from build123d import *

# Parameters (mm, degrees)
SKETCH2_W                = 13
SKETCH2_H                = 21
SKETCH2_W_2              = 12
SKETCH2_H_2              = 20
BOSS_EXTRUDE1_DEPTH      = 3
SKETCH2_2_W              = 12
SKETCH2_2_H              = 20
BOSS_EXTRUDE2_DEPTH      = 3
BOSS_EXTRUDE2_DEPTH_BACK = 5
SKETCH3_W                = 7.910089125
SKETCH3_H                = 16.025972414
SKETCH3_W_2              = 7.710089125
SKETCH3_H_2              = 15.825972414
CUT_EXTRUDE1_DEPTH       = 3
SKETCH3_2_W              = 7.710089125
SKETCH3_2_H              = 15.825972414
BOSS_EXTRUDE3_DEPTH      = 3
CUT_EXTRUDE2_DEPTH       = 11.644897537


with BuildPart() as part:
    # Sketch2 → Boss-Extrude1 (new body)
    with BuildSketch(Plane(origin=(0, 0, 0), x_dir=(1, 0, 0), z_dir=(0, 1, 0))):
        with Locations((-0.268196817, 0.402295225)):
            Rectangle(SKETCH2_W, SKETCH2_H)
        with Locations((-0.268196817, 0.402295225)):
            Rectangle(SKETCH2_W_2, SKETCH2_H_2, mode=Mode.SUBTRACT)
    extrude(amount=BOSS_EXTRUDE1_DEPTH)

    # Sketch2_2 → Boss-Extrude2 (add, two sides)
    with BuildSketch(Plane(origin=(0, 0, 0), x_dir=(1, 0, 0), z_dir=(0, 1, 0))) as boss_extrude2_sk:
        with Locations((-0.268196817, 0.402295225)):
            Rectangle(SKETCH2_2_W, SKETCH2_2_H)
    extrude(amount=BOSS_EXTRUDE2_DEPTH)
    extrude(boss_extrude2_sk.sketch, amount=-BOSS_EXTRUDE2_DEPTH_BACK)

    # Sketch3 → Cut-Extrude1 (cut)
    with BuildSketch(Plane(origin=(0, 3, 0), x_dir=(1, 0, 0), z_dir=(0, 1, 0))):
        with Locations((0.021656158, 0.039979007)):
            Rectangle(SKETCH3_W, SKETCH3_H)
        with Locations((0.021656157, 0.039979007)):
            Rectangle(SKETCH3_W_2, SKETCH3_H_2, mode=Mode.SUBTRACT)
    extrude(amount=-CUT_EXTRUDE1_DEPTH, mode=Mode.SUBTRACT)

    # Sketch3_2 → Boss-Extrude3 (add)
    with BuildSketch(Plane(origin=(0, 3, 0), x_dir=(1, 0, 0), z_dir=(0, 1, 0))):
        with Locations((0.021656157, 0.039979007)):
            Rectangle(SKETCH3_2_W, SKETCH3_2_H)
    extrude(amount=BOSS_EXTRUDE3_DEPTH)

    # Sketch5 → Cut-Extrude2 (cut, through all)
    with BuildSketch(Plane(origin=(3.87670072, 0, 0), x_dir=(0, 0, -1), z_dir=(1, 0, 0))):
        with BuildLine():
            add(Edge.make_bspline(
                [(7.952965214, 3.003696013), (-0.44948354, 3.292111909), (-7.8730072, 5.997516068)],
                knots=[0.001628514, 0.001628514, 0.001628514, 0.990717924, 0.990717924, 0.990717924], degree=2))
            Line((7.952965214, 3.003696013), (7.952965214, 6))
            Line((7.952965214, 6), (-7.8730072, 6))
            Line((-7.8730072, 6), (-7.8730072, 5.997516068))
        make_face()
    extrude(amount=-CUT_EXTRUDE2_DEPTH, mode=Mode.SUBTRACT)


solid = part.part
Source: CAD feature listing. Evaluate the final solid. Frame: model axes, mm. A direction names the side the tool comes from. Give positions to 0.01 mm unless a question says otherwise; leave off trailing zeros. Write each loop counter-clockwise with the first axis right and the second up, starting at its lowest first coordinate (ties: lowest second). Pieces come first, ordered by that corner, then holes. Notation, with made-up numbers: (-36, 2.25) -> (23, 2.25) arc R14 ccw to (23, 21.25) -> close; hole circle Ø1 at (63.25, -8). An arc over 180 degrees is marked (long way). Write item = value, one per line.
Q1. First-contact query: pin 1 (1.5 mm diameter, centred on y = -1.5, z = 0.5, fed in from +X); pin 2 (1 mm diameter, centred on y = -2.5, z = 7.5, fed in from -X); pin 3 (4 mm diameter, centred on x = -1, z = -0.5, fed in from +Y). Flat tips, straight axial feed; report the tip coordinate or a pass-through.
Here are the results:
pin_1 = 5.73
pin_2 = -6.27
pin_3 = 4.16
Q2. Cut plane A-A on y = 1. Return loops of the section in (x, z).
Here are the results:
outline = (-6.77, -10.9) -> (6.23, -10.9) -> (6.23, 10.1) -> (-6.77, 10.1) -> close; (-3.83, -7.95) -> (3.88, -7.95) -> (3.88, 7.87) -> (-3.83, 7.87) -> close; hole (-3.93, -8.05) -> (3.98, -8.05) -> (3.98, 7.97) -> (-3.93, 7.97) -> close
Q3. Cut plane D-D on y = -0.5. Return loops of the section in (x, z).
Here are the results:
outline = (-6.27, -10.4) -> (5.73, -10.4) -> (5.73, 9.6) -> (-6.27, 9.6) -> close
Q4. Reachability of faces 1 (the face through (0, -2, 9.598)), 2 (the face through (-6.268, -2, 0)), 3 (the face through (5.732, -2, 0)) from +Z, -Z, +X, -X, +Y, -Y: full face, straight path, thin tool, end or side. Return the list, or none.
Here are the results:
face_1 = +Z, +X, -X, -Y
face_2 = +Z, -Z, -X, -Y
face_3 = +Z, -Z, +X, -Y
Q5. Line query: line 1 (X direction, y = -2.5, z = 3); line 2 (Y direction, x = -5, z = -2.75); line 3 (Z direction, x = 4.5, y = -0.75). Output: solid intervals per line, ascending. Write a range as from..to.
Here are the results:
line_1 = -6.27..5.73
line_2 = -5..3
line_3 = -10.4..9.6
Q6. Mould query, pull axis Z, two halves, no side actions, for faces 4 (the face through (0, 4, 7.873)), 5 (the face through (0, 1, 10.098)), 6 (the face through (-5, 3, -1)). Classes: +Z half, -Z half, draft (parallel to the pull), parting line (faces both ways), or undercut.
Here are the results:
face_4 = undercut
face_5 = +Z half
face_6 = draft
Q7. Cut plane C-C on z = 8.5. Return loops of the section in (x, y), then the cut area to 3 significant figures.
Here are the results:
outline = (-6.77, 0) -> (-6.27, 0) -> (-6.27, -5) -> (5.73, -5) -> (5.73, 0) -> (6.23, 0) -> (6.23, 3) -> (-6.77, 3) -> close
area = 99.0 mm²
Q8. Cut plane B-B on x = -5.5. Return loops of the section in (y, z).
Here are the results:
outline = (-5, -10.4) -> (0, -10.4) -> (0, -10.9) -> (3, -10.9) -> (3, 10.1) -> (0, 10.1) -> (0, 9.6) -> (-5, 9.6) -> close
